Geometry check sheet. Reference: the model listing, model coordinates, mm. A direction names the side the tool comes from. Round coordinates to 2 decimals unless told otherwise and drop trailing zeros. Write each loop counter-clockwise with the first axis right and the second up, starting at its lowest first coordinate (ties: lowest second). Pieces come first, ordered by that corner, then holes.
Item 1: Cross-section at C-C (x = 66.5). Enter the section's corners in (y, z), then the cut area to 3 significant figures.
Item 2: Cross-section at A-A (z = 30). Enter the section's corners in (x, y).
Item 3: Access from +Z, -Z, +X, -X, +Y, -Y to the whole of each face (thin tool, end or side, straight path). Record for faces 4 (the face through (63, 7, 22)), 5 (the face through (60, 11.5, 37)), 6 (the face through (70, 7, 2)), 7 (the face through (61, 8, 36)), 8 (the face through (10, 7, 35)).
Item 4: Scan lines: probe 1 along X at (y, z) = (6, 4.5); probe 2 along X at (y, z) = (7.25, 30); probe 3 along X at (y, z) = (11, 14). Record each from-to range of solid material in increasing order.
Item 5: Cross-section at B-B (y = 7.5). State how many separate pieces and enclosed holes the cut face has, then the cut area to 3 significant figures.
Item 6: Cross-section at D-D (y = 12.5). Enter the section's corners in (x, z).
Item 7: Depth check by flat-ended pin: P1, Ø2, axis at y = 8.5, z = 34.5, coming from the +X side; P2, Ø6, axis at y = 4, z = 35, coming from the -X side; P3, Ø3.5, axis at x = 4.5, y = 5.5, coming from the +Z side. Enter the tip coordinate at first touch or a pass-through.
Item 8: Draft check along X on faces 1 (the face through (10, 7, 39)), 2 (the face through (0, 7, 2)), 3 (the face through (8, 8, 36)). Enter one of: pulls with the +X half, pulls with the -X half, needs draft (parallel to the pull), parting line crosses it, or undercut.
from build123d import *

# Parameters (mm, degrees)
SKETCH_W        = 70
SKETCH_H        = 15
PAD_DEPTH       = 40
SKETCH001_R     = 25.25
POCKET_DEPTH    = 15
SKETCH002_W     = 7
SKETCH002_H     = 15
POCKET001_DEPTH = 35
SKETCH003_R     = 1.7
POCKET002_DEPTH = 5
SKETCH004_W     = 2
SKETCH004_H     = 8
POCKET003_DEPTH = 11
SKETCH005_W     = 8
SKETCH005_H     = 2
POCKET004_DEPTH = 57
FILLET_R        = 1.9
CHAMFER_SIZE    = 1
FILLET001_R     = 6


with BuildPart() as part:
    # Sketch → Pad (new body)
    with BuildSketch(Plane.XY):
        with Locations((35, 7.5)):
            Rectangle(SKETCH_W, SKETCH_H)
    extrude(amount=PAD_DEPTH)

    # Sketch001 (on Face1 of Pad) → Pocket (cut)
    with BuildSketch(Plane.XZ):
        with Locations((35, 30)):
            Circle(SKETCH001_R)
    extrude(amount=-POCKET_DEPTH, mode=Mode.SUBTRACT)

    # Sketch002 (on Face7 of Pocket) → Pocket001 (cut)
    with BuildSketch(Plane.XY.offset(40)):
        with Locations((3.5, 7.5)):
            Rectangle(SKETCH002_W, SKETCH002_H)
        with Locations((66.5, 7.5)):
            Rectangle(SKETCH002_W, SKETCH002_H)
    extrude(amount=-POCKET001_DEPTH, mode=Mode.SUBTRACT)

    # Sketch003 (on Face11 of Pocket001) → Pocket002 (cut)
    with BuildSketch(Plane.XY.offset(5)):
        with Locations((3.5, 7.5)):
            Circle(SKETCH003_R)
        with Locations((66.5, 7.5)):
            Circle(SKETCH003_R)
    extrude(amount=-POCKET002_DEPTH, mode=Mode.SUBTRACT)

    # Sketch004 (on Face9 of Pocket002) → Pocket003 (cut)
    with BuildSketch(Plane.XY.offset(40)):
        with Locations((11, 7.5)):
            Rectangle(SKETCH004_W, SKETCH004_H)
        with Locations((59, 7.5)):
            Rectangle(SKETCH004_W, SKETCH004_H)
    extrude(amount=-POCKET003_DEPTH, mode=Mode.SUBTRACT)

    # Sketch005 (on Face10 of Pocket003) → Pocket004 (cut)
    with BuildSketch(Plane(origin=(7, 0, 0), x_dir=(0, -1, 0), z_dir=(-1, 0, 0))):
        with Locations((-7.5, 37)):
            Rectangle(SKETCH005_W, SKETCH005_H)
    extrude(amount=-POCKET004_DEPTH, mode=Mode.SUBTRACT)

    # Fillet
    fillet_edges = [part.edges().sort_by_distance(p)[0] for p in [
        (7, 7.5, 40),
        (63, 7.5, 40),
    ]]
    fillet(fillet_edges, radius=FILLET_R)

    # Chamfer
    chamfer_edges = [part.edges().sort_by_distance(p)[0] for p in [
        (1.8, 7.5, 5),
        (64.8, 7.5, 5),
    ]]
    chamfer(chamfer_edges, length=CHAMFER_SIZE)

    # Fillet001
    fillet001_edges = [part.edges().sort_by_distance(p)[0] for p in [
        (0, 0, 2.5),
        (0, 15, 2.5),
        (70, 0, 2.5),
        (70, 15, 2.5),
    ]]
    fillet(fillet001_edges, radius=FILLET001_R)


solid = part.part
Resolved:
1. outline: (0.55, 0) - (5.8, 0) - (5.8, 4) - (4.8, 5) - (0.55, 5) - close; (9.2, 0) - (14.45, 0) - (14.45, 5) - (10.2, 5) - (9.2, 4) - close
1. area: 51.5 mm2
2. outline: (7, 0) - (9.75, 0) - (9.75, 15) - (7, 15) - close; (60.25, 0) - (63, 0) - (63, 15) - (60.25, 15) - close
3. face 4: +Z, +X, +Y, -Y
3. face 5: none
3. face 6: +Z, -Z, +X, +Y, -Y
3. face 7: +X, -X
3. face 8: +Z
4. probe 1: x = 0 to 1.89, 5.11 to 64.89, 68.11 to 70
4. probe 2: x = 7 to 9.75, 60.25 to 63
4. probe 3: x = 7 to 15.47, 54.53 to 63
5. separate pieces: 5
5. enclosed holes: 0
5. area: 758 mm2
6. outline: (1.13, 0) - (68.87, 0) - (68.87, 5) - (63, 5) - (63, 38.1) arc R1.9 ccw to (61.1, 40) - (58.19, 40) arc R25.25 cw (long way) to (11.81, 40) - (8.9, 40) arc R1.9 ccw to (7, 38.1) - (7, 5) - (1.13, 5) - close
7. P1: stops at x = 63
7. P2: stops at x = 7
7. P3: stops at z = 5
8. face 1: undercut
8. face 2: pulls with the -X half
8. face 3: needs draft
